Build history of the part. All positions in model axes, mm. A direction names the side the tool comes from. Give positions to 0.01 mm unless a question says otherwise; leave off trailing zeros. Write each loop counter-clockwise with the first axis right and the second up, starting at its lowest first coordinate (ties: lowest second). Pieces come first, ordered by that corner, then holes. Notation, with made-up numbers: M 40,26 L 47,26 A10 ccw 47,34 Z; hole C 43,81.25 d4. An arc over 180 degrees is marked long. One line per item, written item: value. Start each with the question number.
from build123d import *

# Parameters (mm, degrees)
F1_DEPTH  = 631.5
F2_DEPTH  = 70.75
F3_W      = 10.45
F3_H      = 70.75
F4_DEPTH  = 620
F5_W      = 450
F5_H      = 80.75
F6_DEPTH  = 25.4
F7_R      = 4.99999
F9_DEPTH  = 631.5
F10_DEPTH = 70.75
F11_W     = 10.45
F11_H     = 70.75
F12_DEPTH = 620
F13_W     = 12.75
F13_H     = 101.2
F14_DEPTH = 631.5
F16_DEPTH = 631.5
F18_DEPTH = 300
F19_DEPTH = 300


# Not quite as in the source:
# - a fillet or chamfer is up to 0.001 mm smaller than in the source, because OpenCascade refuses the exact size


with BuildPart() as f1:
    # F0 (on Front) → F1 (new body)
    with BuildSketch(Plane.XZ):
        Polygon((0, 38.1), (0, 31.75), (31.75, 31.75), (31.75, 0), (38.1, 0), (38.1, 38.1), align=None)
    extrude(amount=F1_DEPTH)

    # F0 (on Front) → F2 (join)
    with BuildSketch(Plane.XZ):
        Polygon((-10.45, 0), (0, 0), (0, 31.75), (0, 38.1), (0, 620), (-10.45, 620), align=None)
    extrude(amount=F2_DEPTH)

    # F3 (on Top) → F4 (join)
    with BuildSketch(Plane.XY):
        with Locations((-5.225, -596.125)):
            Rectangle(F3_W, F3_H)
    extrude(amount=F4_DEPTH)

    # F5 (on Top) → F6 (join)
    with BuildSketch(Plane.XY):
        with Locations((67.2, -35.375)):
            Rectangle(F5_W, F5_H)
        with Locations((67.2, -596.125)):
            Rectangle(F5_W, F5_H)
    extrude(amount=-F6_DEPTH)

    # F7 (radius 5 in the source; OpenCascade refuses exactly that, so slightly less here)
    f7_edges = [f1.edges().sort_by_distance(p)[0] for p in [
        (67.2, -636.5, 0),
        (165.15, -555.75, 0),
        (165.15, -75.75, 0),
        (67.2, 5, 0),
        (-63.025, -75.75, 0),
        (-63.025, -555.75, 0),
    ]]
    fillet(f7_edges, radius=F7_R)

    # F8 (on Front) → F9 (join)
    with BuildSketch(Plane.XZ):
        Polygon((102.65, 31.75), (134.4, 31.75), (134.4, 38.1), (96.3, 38.1), (96.3, 0), (102.65, 0), align=None)
    extrude(amount=F9_DEPTH)

    # F8 (on Front) → F10 (join)
    with BuildSketch(Plane.XZ):
        Polygon((134.4, 31.75), (134.4, 0), (144.85, 0), (144.85, 620), (134.4, 620), (134.4, 38.1), align=None)
        Polygon((102.65, 31.75), (134.4, 31.75), (134.4, 38.1), (96.3, 38.1), (96.3, 0), (102.65, 0), align=None)
    extrude(amount=F10_DEPTH)

    # F11 (on Top) → F12 (join)
    with BuildSketch(Plane.XY):
        with Locations((139.625, -596.125)):
            Rectangle(F11_W, F11_H)
    extrude(amount=F12_DEPTH)

    # F13 (on Front) → F14 (join)
    with BuildSketch(Plane.XZ):
        with Locations((-16.825, 569.4)):
            Rectangle(F13_W, F13_H)
        with Locations((151.225, 569.4)):
            Rectangle(F13_W, F13_H)
    extrude(amount=F14_DEPTH)

    # F15 (on Front) → F16 (join)
    with BuildSketch(Plane.XZ):
        Polygon((-48.55, 4.763), (-48.55, 0), (-10.45, 0), (-10.45, 38.1), (-15.213, 38.1), (-15.213, 4.763), align=None)
        Polygon((144.85, 0), (182.95, 0), (182.95, 4.763), (149.613, 4.763), (149.613, 38.1), (144.85, 38.1), align=None)
    extrude(amount=F16_DEPTH)

    # F17 (on Right) → F18 (cut)
    with BuildSketch(Plane.YZ):
        with BuildLine():
            Line((-631.5, -10), (-631.5, -25.4))
            Line((-631.5, -25.4), (-560.75, -25.4))
            Line((-560.75, -25.4), (-560.75, -10))
            ThreePointArc((-560.75, -10), (-562.2144660941, -6.4644660941), (-565.75, -5))
            Line((-565.75, -5), (-626.5, -5))
            ThreePointArc((-626.5, -5), (-630.0355339059, -6.4644660941), (-631.5, -10))
        make_face()
        with BuildLine():
            Line((-5, -5), (-65.75, -5))
            ThreePointArc((-65.75, -5), (-69.2855339059, -6.4644660941), (-70.75, -10))
            Line((-70.75, -10), (-70.75, -25.4))
            Line((-70.75, -25.4), (0, -25.4))
            Line((0, -25.4), (0, -10))
            ThreePointArc((0, -10), (-1.4644660941, -6.4644660941), (-5, -5))
        make_face()
    extrude(amount=F18_DEPTH, mode=Mode.SUBTRACT)

    # F17 (on Right) → F19 (cut)
    with BuildSketch(Plane.YZ):
        with BuildLine():
            Line((-631.5, -10), (-631.5, -25.4))
            Line((-631.5, -25.4), (-560.75, -25.4))
            Line((-560.75, -25.4), (-560.75, -10))
            ThreePointArc((-560.75, -10), (-562.2144660941, -6.4644660941), (-565.75, -5))
            Line((-565.75, -5), (-626.5, -5))
            ThreePointArc((-626.5, -5), (-630.0355339059, -6.4644660941), (-631.5, -10))
        make_face()
        with BuildLine():
            Line((-5, -5), (-65.75, -5))
            ThreePointArc((-65.75, -5), (-69.2855339059, -6.4644660941), (-70.75, -10))
            Line((-70.75, -10), (-70.75, -25.4))
            Line((-70.75, -25.4), (0, -25.4))
            Line((0, -25.4), (0, -10))
            ThreePointArc((0, -10), (-1.4644660941, -6.4644660941), (-5, -5))
        make_face()
    extrude(amount=-F19_DEPTH, mode=Mode.SUBTRACT)


solid = f1.part
1) Drop flat-ended pins along their axis: P1, Ø16, axis at x = 126, y = -163.5, coming from the -Z side; P2, Ø3, axis at x = 34, y = -401, coming from the -Z side; P3, Ø5, axis at x = -7.5, z = 185.5, coming from the -Y side. Give the stop position or say it passes through.
2) Band-saw the part on C-C (x = 244.5). List the corners of the cut face in (y, z).
3) Probe line 1 along X through (y, z) = (-457.5, 572); line 2 along X through (y, z) = (-598.5, 232); line 3 along Z through (x, y) = (138, -582.5). List the from-to ranges inside material, lowest first. Write a range as from..to.
4) Band-saw the part on B-B (y = -356). Count the separate pieces of the cut face and the enclosed holes in it, then the cut area to 3 significant figures.
5) Mould opens along X. For faces 5 (the face through (64, -636.5, -15)), 6 (the face through (144.85, -312, 19)) say: released by +X, released by -X, zero draft, split by the parting line, or undercut.
6) Band-saw the part on A-A (z = 112.5). List the corners of the cut face in (x, y).
7) Tool access for faces 1 (the face through (19, -311, 38.1)), 2 (the face through (143, 0, 311)), 3 (the face through (70, -70.75, -18)), 4 (the face through (64, -596, 0)): list every direction of +Z, -Z, +X, -X, +Y, -Y with a clear straight run to the whole face (end or side of a thin tool).
Model answer:
1. P1: stops at z = 31.75
1. P2: stops at z = 0
1. P3: stops at y = -631.5
2. outline: M -636.5,-25.4 L -631.5,-25.4 L -631.5,-10 A5 cw -626.5,-5 L -565.75,-5 A5 cw -560.75,-10 L -560.75,-25.4 L -555.75,-25.4 L -555.75,-5 A5 ccw -560.75,0 L -631.5,0 A5 ccw -636.5,-5 Z; M -75.75,-25.4 L -70.75,-25.4 L -70.75,-10 A5 cw -65.75,-5 L -5,-5 A5 cw 0,-10 L 0,-25.4 L 5,-25.4 L 5,-5 A5 ccw 0,0 L -70.75,0 A5 ccw -75.75,-5 Z
3. line 1: x = -23.2..-10.45, 144.85..157.6
3. line 2: x = -10.45..0, 134.4..144.85
3. line 3: z = -5..620
4. separate pieces: 6
4. enclosed holes: 0
4. area: 4,150 mm²
5. face 5: zero draft
5. face 6: undercut
6. outline: M -10.45,-631.5 L 0,-631.5 L 0,-560.75 L -10.45,-560.75 Z; M -10.45,-70.75 L 0,-70.75 L 0,0 L -10.45,0 Z; M 134.4,-631.5 L 144.85,-631.5 L 144.85,-560.75 L 134.4,-560.75 Z; M 134.4,-70.75 L 144.85,-70.75 L 144.85,0 L 134.4,0 Z
7. face 1: +Z, +Y, -Y
7. face 2: +Z, +X, -X, +Y
7. face 3: -Z, +X, -X
7. face 4: +Z, +Y, -Y
